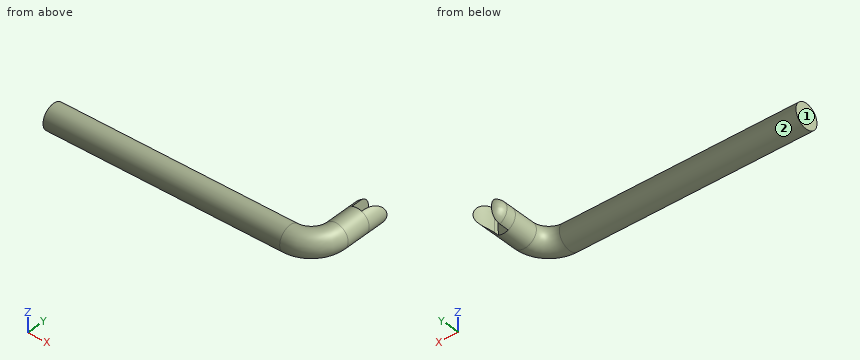
from build123d import *

# Parameters (mm, degrees)
SKETCH1_R                      = 3.175
BOSS_EXTRUDE1_START            = 5.08
BOSS_EXTRUDE1_DEPTH            = 5.08
BOSS_EXTRUDE2_REACH            = 74.32
BOSS_EXTRUDE2_END_MAJOR_RADIUS = 92.053833851
BOSS_EXTRUDE2_END_MINOR_RADIUS = 6.985
FILLET1_R                      = 2.54


with BuildPart() as part:
    # Sweep3: sweep along a path in Sketch2
    with BuildLine(Plane.XY) as sweep3_path:
        Line((0, 0), (60.96, 0))
        ThreePointArc((60.96, 0), (65.450128061, 1.859871939), (67.31, 6.35))
        Line((67.31, 6.35), (67.31, 12.7))
    # Sketch1 → Sweep3 (sweep)
    with BuildSketch(Plane(origin=(0, 0, 0), x_dir=(0, 0, -1), z_dir=(1, 0, 0))):
        Circle(SKETCH1_R)
    sweep(path=sweep3_path.line)

    # Sketch3 → Boss-Extrude1 (add)
    with BuildSketch(Plane(origin=(0, 12.7, 0), x_dir=(1, 0, 0), z_dir=(0, 1, 0)).offset(BOSS_EXTRUDE1_START)):
        with BuildLine():
            ThreePointArc((65.989488636, 2.88736467), (64.135, 0), (65.989488636, -2.88736467))
            ThreePointArc((65.989488636, -2.88736467), (66.04, 0), (65.989488636, 2.88736467))
        make_face()
    extrude(amount=-BOSS_EXTRUDE1_DEPTH)

    # Boss-Extrude2: up to this torus (the profile starts inside it)
    boss_extrude2_end = Plane(origin=(-16.51, 13.243362772, 0), z_dir=(0, -1, 0)) * Torus(BOSS_EXTRUDE2_END_MAJOR_RADIUS, BOSS_EXTRUDE2_END_MINOR_RADIUS, mode=Mode.PRIVATE)
    # Sketch4 → Boss-Extrude2 (add, up to the surface)
    with BuildSketch(Plane(origin=(0, 12.7, 0), x_dir=(1, 0, 0), z_dir=(0, 1, 0)), mode=Mode.PRIVATE) as boss_extrude2_sk1:
        with BuildLine():
            ThreePointArc((68.529488636, -2.931462513), (70.485, 0), (68.529488636, 2.931462513))
            ThreePointArc((68.529488636, 2.931462513), (68.58, 0), (68.529488636, -2.931462513))
        make_face()
    boss_extrude2_tool1 = extrude(boss_extrude2_sk1.sketch, amount=BOSS_EXTRUDE2_REACH, mode=Mode.PRIVATE) & boss_extrude2_end
    add(boss_extrude2_tool1.solids().sort_by_distance((69.356115, 12.7, 0))[0])

    # Fillet1
    # the kernel refuses this fillet: 2.54 mm, written as the material it takes off along each edge
    with BuildSketch(Plane(origin=(67.31, 17.78, 0), x_dir=(0.9999950652018583, 0, -0.0031415874858765833), z_dir=(0.0031415874858765833, 0, 0.9999950652018583))) as fillet1_piece_1_section:
        with BuildLine():
            CenterArc((3.175 - FILLET1_R, -FILLET1_R), FILLET1_R, 0, 90)
            Line((3.175 - FILLET1_R, 0), (3.175, 0))
            Line((3.175, 0), (3.175, -FILLET1_R))
        make_face()
    fillet1_piece_1 = revolve(axis=Axis((67.31, 17.78, 0), (0, 1, 0)), revolution_arc=359.64, mode=Mode.PRIVATE)
    fillet1_piece_1 = fillet1_piece_1 & Plane(origin=(-16.51, 16.807436712, 0), x_dir=(0.9993881118881123, 0, 0.03497716135872228), z_dir=(0, 1, 0)) * Cylinder(82.55, 13, mode=Mode.PRIVATE)
    add(fillet1_piece_1, mode=Mode.SUBTRACT)


solid = part.part
Could you check a few things on this model? Use its own coordinates, in mm. Face numbers are marked on the shaded views. A direction names the side the tool comes from. Give positions to 0.01 mm unless a question says otherwise; leave off trailing zeros. Order: outer loops, then holes, each group sorted by start corner. A loop starts at its lowest first (then second) coordinate and runs counter-clockwise, first axis right, second up.
1. Will these pins go through, and if not, where does the flat tip stop? P1, Ø5, axis at x = 41.5, y = 3.5, coming from the -Z side; P2, Ø4, axis at x = 62.5, y = 6, coming from the -Z side.
2. Suppose I cut it at B-B (x = 60). List the corners of the cut face in (y, z) for me (3 decimals).
3. Suppose I cut it at A-A (y = 12). List the corners of the cut face in (x, z) for me (3 decimals), plus the area to 3 significant figures.
4. I need wall thicknesses on L1, parallel to Y at x = 50, z = 0.25; L2, parallel to X at y = 14, z = -2; L3, parallel to X at y = -1.75, z = 2. Which ranges of each line are inside material? Lowest first, please.
5. For the marked faces 1 and 2, which set-ups out of +Z, -Z, +X, -X, +Y, -Y let a thin tool reach every point of the face, with its end or its side?
Solved:
1. P1: stops at z = -3.01
1. P2: stops at z = -1.55
2. outline: circle Ø6.35 at (0, 0)
3. outline: circle Ø6.35 at (67.31, 0)
3. area: 31.7 mm2
4. L1: y = -3.17 to 3.17
4. L2: x = 64.84 to 66.02, 68.58 to 69.78
4. L3: x = 0 to 64.44
5. face 1: +Z, -Z, -X, +Y, -Y
5. face 2: -X
